Source: three-view drawing plus pictorial views. Frame: mm from the lowest corner of the part. Coordinates: 2 decimals unless noted, no trailing zeros. Order: outer loops, then holes, each group sorted by start corner. A loop starts at its lowest first (then second) coordinate and runs counter-clockwise, first axis right, second up. Notation, with made-up numbers: M 20.5,70.5 L 71.5,70.5 A31 ccw 71.5,107.5 Z; hole C 38,66 d6. An arc over 180 degrees is marked long. Write item = value, one per line. Start each with the question number.
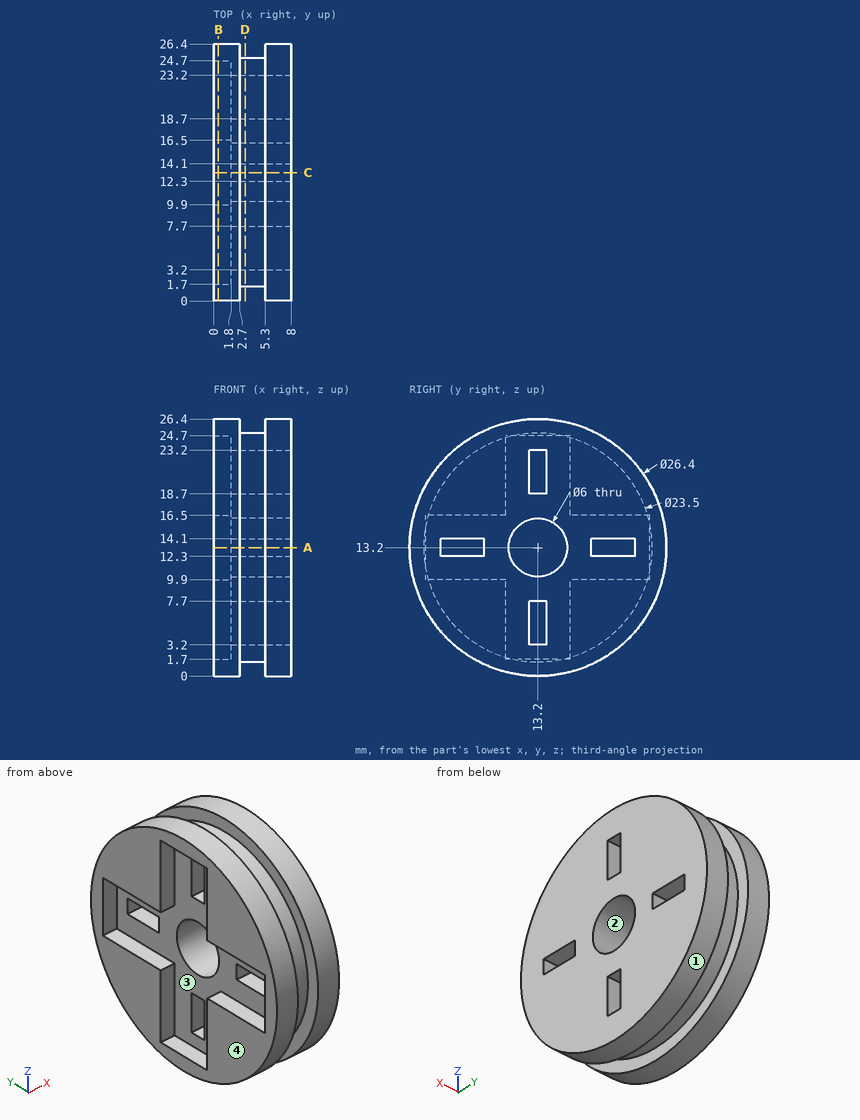
Item 1: Section query D-D on x = 3.25. Output: boundary loops of the cut face in (y, z), and give its area (3 significant figures).
Item 2: Section query A-A on z = 13.2. Output: boundary loops of the cut face in (x, y), and give its area (3 significant figures).
Item 3: Draft query along Y for the marked faces 1, 2, 3 and 4. Return one class per face: pulls with the +Y half, pulls with the -Y half, needs draft (parallel to the pull), parting line crosses it, or undercut.
Item 4: Section query B-B on x = 0.5. Output: boundary loops of the cut face in (y, z), and give its area (3 significant figures).
Item 5: Material intervals for probe 1 along Y at (x, z) = (5.25, 13.2); probe 2 along Z at (x, y) = (2.75, 13); probe 3 along Y at (x, z) = (6.25, 13.2), sorted ascending. Write a range as [from, to].
Item 6: First-contact query: pin 1 (4 mm diameter, centred on x = 6, y = 19.5, fed in from -Z); pin 2 (2 mm diameter, centred on x = 4, z = 6, fed in from +Y); pin 3 (1 mm diameter, centred on x = 6, z = 19, fed in from -Y). Flat tips, straight axial feed; report the tip coordinate or a pass-through.
Ans:
q1.outline = C 13.2,13.2 d23.5; hole M 3.2,12.3 L 7.7,12.3 L 7.7,14.1 L 3.2,14.1 Z; hole C 13.2,13.2 d6; hole M 12.3,3.2 L 14.1,3.2 L 14.1,7.7 L 12.3,7.7 Z; hole M 12.3,18.7 L 14.1,18.7 L 14.1,23.2 L 12.3,23.2 Z; hole M 18.7,12.3 L 23.2,12.3 L 23.2,14.1 L 18.7,14.1 Z
q1.area = 373 mm^2
q2.outline = M 0,0 L 2.7,0 L 2.7,1.45 L 5.3,1.45 L 5.3,0 L 8,0 L 8,3.2 L 1.8,3.2 L 1.8,1.7 L 0,1.7 Z; M 0,24.7 L 1.8,24.7 L 1.8,23.2 L 8,23.2 L 8,26.4 L 5.3,26.4 L 5.3,24.95 L 2.7,24.95 L 2.7,26.4 L 0,26.4 Z; M 1.8,7.7 L 8,7.7 L 8,10.2 L 1.8,10.2 Z; M 1.8,16.2 L 8,16.2 L 8,18.7 L 1.8,18.7 Z
q2.area = 69.3 mm^2
q3.face_1 = parting line crosses it
q3.face_2 = undercut
q3.face_3 = undercut
q3.face_4 = needs draft
q4.outline = C 13.2,13.2 d26.4; hole M 1.7,9.9 L 9.9,9.9 L 9.9,1.7 L 16.5,1.7 L 16.5,9.9 L 24.7,9.9 L 24.7,16.5 L 16.5,16.5 L 16.5,24.7 L 9.9,24.7 L 9.9,16.5 L 1.7,16.5 Z
q4.area = 287 mm^2
q5.probe_1 = [1.45, 3.2], [7.7, 10.2], [16.2, 18.7], [23.2, 24.95]
q5.probe_2 = [1.45, 3.2], [7.7, 10.21], [16.19, 18.7], [23.2, 24.95]
q5.probe_3 = [0, 3.2], [7.7, 10.2], [16.2, 18.7], [23.2, 26.4]
q6.pin_1 = 0.72
q6.pin_2 = 23.18
q6.pin_3 = 1.11
